from build123d import *

# Parameters (mm, degrees)
ARRAY_X_COUNT = 3
ARRAY_X_PITCH = 18
ARRAY_Y_COUNT = 3
ARRAY_Y_PITCH = 18
BOX_W         = 56
BOX_H         = 56
BOX_DEPTH     = 10


with BuildPart() as array:
    # Sphere → Sphere (revolve)
    with BuildSketch(Plane.XZ):
        with BuildLine():
            ThreePointArc((0, -5), (5, 0), (0, 5))
            Line((0, 5), (0, -5))
        make_face()
    revolve(axis=Axis((0, 0, 0), (0, 0, 1)))

    # Array X: Array ×3


with BuildPart() as array_1:
    add(array.part)
    with Locations(*[(i * ARRAY_X_PITCH, 0, 0) for i in range(1, ARRAY_X_COUNT)]):
        add(array.part)

    # Array Y: Array ×3


with BuildPart() as array_2:
    add(array_1.part)
    with Locations(*[(0, i * ARRAY_Y_PITCH, 0) for i in range(1, ARRAY_Y_COUNT)]):
        add(array_1.part)


with BuildPart() as cut:
    # Box → Box (new body)
    with BuildSketch(Plane(origin=(-10, -10, -10), x_dir=(1, 0, 0), z_dir=(0, 0, 1))):
        with Locations((28, 28)):
            Rectangle(BOX_W, BOX_H)
    extrude(amount=BOX_DEPTH)

    # Cut: cut Array
    add(array_2.part, mode=Mode.SUBTRACT)


solid = cut.part
For this review, take the finished solid that the model builds, in its own axes (mm). Give positions to 0.01 mm unless a question says otherwise; leave off trailing zeros. Loops run counter-clockwise (first coordinate to the right, second up) from the corner with the lowest first, then second, coordinate; pieces in that order, holes last.
Item 1: Take a section at C-C, the plane y = 35. State the section outline as (x, z) points, and give its area (3 significant figures).
Item 2: Insertion check: pin 1 (6 mm diameter, centred on x = 11.5, y = 26, fed in from +Z). The pin has a flat end and moves straight along its axis. Give the tip position at first contact, or say it passes through.
Item 3: Take a section at A-A, the plane x = -3. State the section outline as (y, z) points, and give its area (3 significant figures).
Item 4: For line 1 along Y through (x, z) = (37, -3.5); line 2 along X through (y, z) = (37, -1.5), list the stretches that pass through material, from the lowest coordinate up.
Item 5: Take a section at B-B, the plane z = -2.75. Give the number of separate pieces and of enclosed holes in the cut face, and give its area (3 significant figures).
Calculated:
1. outline: (-10, -10) - (46, -10) - (46, 0) - (40.9, 0) arc R4.9 cw to (31.1, 0) - (22.9, 0) arc R4.9 cw to (13.1, 0) - (4.9, 0) arc R4.9 cw to (-4.9, 0) - (-10, 0) - close
1. area: 447 mm2
2. pin 1: stops at z = 0
3. outline: (-10, -10) - (46, -10) - (46, 0) - (40, 0) arc R4 cw to (32, 0) - (22, 0) arc R4 cw to (14, 0) - (4, 0) arc R4 cw to (-4, 0) - (-10, 0) - close
3. area: 485 mm2
4. line 1: y = -10 to -3.43, 3.43 to 14.57, 21.43 to 32.57, 39.43 to 46
4. line 2: x = -10 to -4.66, 4.66 to 13.34, 22.66 to 31.34, 40.66 to 46
5. separate pieces: 1
5. enclosed holes: 9
5. area: 2,640 mm2
